```python
from build123d import *

# Parameters (mm, degrees)
SKETCH_1_W          = 80.5
SKETCH_1_H          = 60.5
EXTRUDE_1_DEPTH     = 1.5
SKETCH_2_W          = 76.3
SKETCH_2_H          = 56.3
SKETCH_2_W_2        = 73.3
SKETCH_2_H_2        = 53.3
EXTRUDE_2_DEPTH     = 4
SKETCH_4_W          = 2
SKETCH_4_H          = 35.5
SKETCH_4_H_2        = 42
CUT_EXTRUDE_1_DEPTH = 4
SKETCH_5_R          = 1.8
SKETCH_5_R_2        = 2.5
CUT_EXTRUDE_2_DEPTH = 3


with BuildPart() as part:
    # 草图1 → 凸台-拉伸1 (new body)
    with BuildSketch(Plane(origin=(0, 0, 0), x_dir=(1, 0, 0), z_dir=(0, 1, 0))):
        Rectangle(SKETCH_1_W, SKETCH_1_H)
    extrude(amount=EXTRUDE_1_DEPTH)

    # 草图2 → 凸台-拉伸2 (add)
    with BuildSketch(Plane(origin=(0, 1.5, 0), x_dir=(1, 0, 0), z_dir=(0, 1, 0))):
        Rectangle(SKETCH_2_W, SKETCH_2_H)
        Rectangle(SKETCH_2_W_2, SKETCH_2_H_2, mode=Mode.SUBTRACT)
    extrude(amount=EXTRUDE_2_DEPTH)

    # 草图4 → 切除-拉伸1 (cut)
    with BuildSketch(Plane(origin=(0, 5.5, 0), x_dir=(1, 0, 0), z_dir=(0, 1, 0))):
        with Locations((37.4, -1.4)):
            Rectangle(SKETCH_4_W, SKETCH_4_H)
        with Locations((-37.4, 0.35)):
            Rectangle(SKETCH_4_W, SKETCH_4_H_2)
    extrude(amount=-CUT_EXTRUDE_1_DEPTH, mode=Mode.SUBTRACT)

    # 草图5 → 切除-拉伸2 (cut)
    with BuildSketch(Plane.XZ):
        with Locations((20.35, -22.75)):
            Circle(SKETCH_5_R)
        with Locations((27.45, -22.75)):
            Circle(SKETCH_5_R)
        with Locations((-10.15, 17.15)):
            Circle(SKETCH_5_R_2)
    extrude(amount=-CUT_EXTRUDE_2_DEPTH, mode=Mode.SUBTRACT)


solid = part.part
```
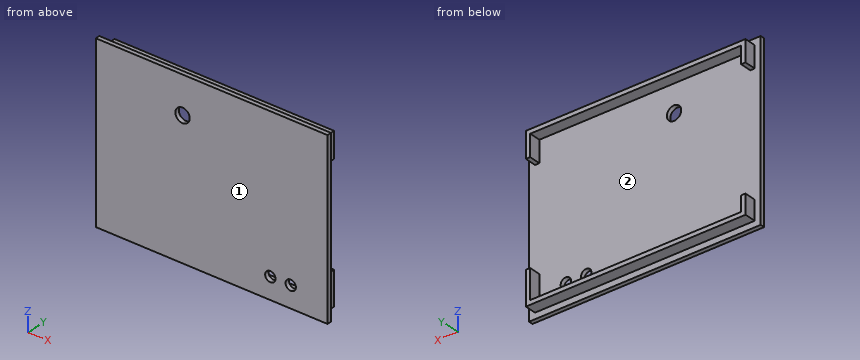
Input: part model. Units: mm. Frame: model coordinates. Face numbers are marked on the shaded views. Round coordinates to 2 decimals unless told otherwise and drop trailing zeros. Write each loop counter-clockwise with the first axis right and the second up, starting at its lowest first coordinate (ties: lowest second). Pieces come first, ordered by that corner, then holes. Notation, with made-up numbers: M -25.75,33.5 L -13.75,33.5 A12 cw -13.75,44.5 Z; hole C -16.75,44.5 d8. An arc over 180 degrees is marked long. Write each question's results on one line, items separated by ' | '.
Q1. Line query: line 1 along Z through (x, y) = (27.45, 0.75); line 2 along Z through (x, y) = (-10.15, 1.1); line 3 along X through (y, z) = (3.2, -21.5). Output: solid intervals per line, ascending.
Results:
line 1: z = -30.25 to -24.55, -20.95 to 30.25 | line 2: z = -30.25 to 14.65, 19.65 to 30.25 | line 3: x = -38.15 to -36.65, 36.65 to 38.15
Q2. Section query B-B (z = 17.15). Return loops of the section in (x, y), and give its area (3 significant figures).
Results:
outline: M -40.25,0 L -12.65,0 L -12.65,1.5 L -40.25,1.5 Z; M -7.65,0 L 40.25,0 L 40.25,1.5 L -7.65,1.5 Z | area: 113 mm^2
Q3. Draft query along Z for the marked faces 1 and 2. Return one class per face: released by +Z, released by -Z, zero draft, split by the parting line, or undercut.
Results:
face 1: zero draft | face 2: undercut
Q4. Pin query (flat end, axial travel): P1, Ø1, axis at x = -9, y = 2.5, coming from the -Z side; P2, Ø2, axis at x = -23.5, y = 5, coming from the +Z side; P3, Ø1.2, axis at y = 4, z = -21, coming from the -X side. Return the tip coordinate at first contact, or that it passes through.
Results:
P1: stops at z = -28.15 | P2: stops at z = 28.15 | P3: stops at x = -38.15
Q5. Section query C-C (z = -22.75). Return loops of the section in (x, y).
Results:
outline: M -40.25,0 L 18.55,0 L 18.55,1.5 L -36.65,1.5 L -36.65,5.5 L -38.15,5.5 L -38.15,1.5 L -40.25,1.5 Z; M 22.15,0 L 25.65,0 L 25.65,1.5 L 22.15,1.5 Z; M 29.25,0 L 40.25,0 L 40.25,1.5 L 38.15,1.5 L 38.15,5.5 L 36.65,5.5 L 36.65,1.5 L 29.25,1.5 Z
Q6. Section query D-D (y = 3.95). Return loops of the section in (x, z), and give its area (3 significant figures).
Results:
outline: M -38.15,-28.15 L 38.15,-28.15 L 38.15,-16.35 L 36.65,-16.35 L 36.65,-26.65 L -36.65,-26.65 L -36.65,-21.35 L -38.15,-21.35 Z; M -38.15,20.65 L -36.65,20.65 L -36.65,26.65 L 36.65,26.65 L 36.65,19.15 L 38.15,19.15 L 38.15,28.15 L -38.15,28.15 Z | area: 273 mm^2
Q7. Section query A-A (x = 27.45). Return loops of the section in (y, z).
Results:
outline: M 0,-30.25 L 1.5,-30.25 L 1.5,-28.15 L 5.5,-28.15 L 5.5,-26.65 L 1.5,-26.65 L 1.5,-24.55 L 0,-24.55 Z; M 0,-20.95 L 1.5,-20.95 L 1.5,26.65 L 5.5,26.65 L 5.5,28.15 L 1.5,28.15 L 1.5,30.25 L 0,30.25 Z
